from build123d import *

# Parameters (mm, degrees)
SKETCH1_W           = 260
SKETCH1_H           = 350
BOSS_EXTRUDE1_DEPTH = 54
FILLET1_R           = 54


with BuildPart() as part:
    # Sketch1 → Boss-Extrude1 (new body)
    with BuildSketch(Plane.XY):
        Rectangle(SKETCH1_W, SKETCH1_H)
    extrude(amount=BOSS_EXTRUDE1_DEPTH)

    # Fillet1
    fillet1_edges = [part.edges().sort_by_distance(p)[0] for p in [
        (130, 0, 54),
        (-130, 0, 54),
        (0, -175, 54),
        (0, 175, 54),
    ]]
    fillet(fillet1_edges, radius=FILLET1_R - 0.0001)  # a hair under: the kernel refuses the full size


solid = part.part
Source: CAD feature listing. Evaluate the final solid. Frame: model axes, mm. Round coordinates to 2 decimals unless told otherwise and drop trailing zeros. Write each loop counter-clockwise with the first axis right and the second up, starting at its lowest first coordinate (ties: lowest second). Pieces come first, ordered by that corner, then holes. Notation, with made-up numbers: M 76.25,28 L 90.25,28 A30 ccw 90.25,62 Z; hole C -34.75,-25.5 d10. An arc over 180 degrees is marked long. One line per item, written item: value. Start each with the question number.
Item 1: Section query D-D (z = 14). Return the cut outline in (x, y).
Item 2: Section query C-C (z = 38). Return the cut outline in (x, y).
Item 3: Ray query, L1, parallel to Y at x = 90, z = 3; L2, parallel to Y at x = 45.5, z = 7; L3, parallel to Z at x = -24.5, y = 161. Return the intervals inside material, ascending. Write a range as from..to.
Item 4: Pin query (flat end, axial travel): pin 1 (1.5 mm diameter, centred on y = -137, z = 29.5, fed in from -X); pin 2 (4 mm diameter, centred on y = 28, z = 35, fed in from -X); pin 3 (6 mm diameter, centred on y = 122.5, z = 7.5, fed in from -X). Return the tip coordinate at first contact, or that it passes through.
Result set:
1. outline: M -128.15,-173.15 L 128.15,-173.15 L 128.15,173.15 L -128.15,173.15 Z
2. outline: M -114.37,-159.37 L 114.37,-159.37 L 114.37,159.37 L -114.37,159.37 Z
3. L1: y = -174.92..174.92
3. L2: y = -174.54..174.54
3. L3: z = 0..36.28
4. pin 1: stops at x = -121.71
4. pin 2: stops at x = -118.74
4. pin 3: stops at x = -129.81
